from build123d import *

# Parameters (mm, degrees)
SKETCH_1_W          = 20
SKETCH_1_H          = 20
SKETCH_1_W_2        = 18
SKETCH_1_H_2        = 18
EXTRUDE_1_DEPTH     = 396
SKETCH_2_R          = 1.45
CUT_EXTRUDE_1_DEPTH = 397.630810704
SKETCH_3_R          = 1.45
CUT_EXTRUDE_2_DEPTH = 397.630810704


with BuildPart() as part:
    # 草图1 → 凸台-拉伸1 (new body)
    with BuildSketch(Plane(origin=(0, 0, 0), x_dir=(0, 0, -1), z_dir=(1, 0, 0))):
        Rectangle(SKETCH_1_W, SKETCH_1_H)
        Rectangle(SKETCH_1_W_2, SKETCH_1_H_2, mode=Mode.SUBTRACT)
    extrude(amount=EXTRUDE_1_DEPTH)

    # 草图2 → 切除-拉伸1 (cut, through all)
    with BuildSketch(Plane(origin=(0, 0, -10), x_dir=(-1, 0, 0), z_dir=(0, 0, -1))):
        with Locations((-380, -12.5)):
            Circle(SKETCH_2_R)
        with Locations(Location((-390.825317547, -6.25, 0), (0, 0, 90))):
            Circle(SKETCH_2_R)
        with Locations(Location((-390.825317547, 6.25, 0), (0, 0, 90))):
            Circle(SKETCH_2_R)
        with Locations((-380, 12.5)):
            Circle(SKETCH_2_R)
        with Locations(Location((-369.174682453, 6.25, 0), (0, 0, 90))):
            Circle(SKETCH_2_R)
        with Locations(Location((-369.174682453, -6.25, 0), (0, 0, 90))):
            Circle(SKETCH_2_R)
        with Locations(Location((-380, 0, 0), (0, 0, 90))):
            Circle(SKETCH_2_R)
    extrude(amount=-CUT_EXTRUDE_1_DEPTH, mode=Mode.SUBTRACT)

    # 草图3 → 切除-拉伸2 (cut, through all)
    with BuildSketch(Plane.XY.offset(10)):
        with Locations((10, 5)):
            Circle(SKETCH_3_R)
        with Locations((20, 5)):
            Circle(SKETCH_3_R)
        with Locations((10, -5)):
            Circle(SKETCH_3_R)
        with Locations((20, -5)):
            Circle(SKETCH_3_R)
        with Locations(Location((369.174682453, 6.25, 0), (0, 0, 90))):
            Circle(SKETCH_3_R)
        with Locations(Location((380, 0, 0), (0, 0, 90))):
            Circle(SKETCH_3_R)
        with Locations(Location((369.174682453, -6.25, 0), (0, 0, 90))):
            Circle(SKETCH_3_R)
        with Locations(Location((390.825317547, -6.25, 0), (0, 0, 90))):
            Circle(SKETCH_3_R)
        with Locations(Location((390.825317547, 6.25, 0), (0, 0, 90))):
            Circle(SKETCH_3_R)
    extrude(amount=-CUT_EXTRUDE_2_DEPTH, mode=Mode.SUBTRACT)


solid = part.part
Can you work these out from the model? Positions are in its coordinate system, mm. A direction names the side the tool comes from. Give positions to 0.01 mm unless a question says otherwise; leave off trailing zeros. Loops run counter-clockwise (first coordinate to the right, second up) from the corner with the lowest first, then second, coordinate; pieces in that order, holes last. Notation, with made-up numbers: (87, -0.5) -> (92, -0.5) arc R11 ccw to (92, 17.5) -> close; hole circle Ø9 at (64, 40.5). An arc over 180 degrees is marked (long way). Write item = value, one per line.
1) Will this pin go through, and if not, where does the flat tip stop? pin 1 (2.5 mm diameter, centred on x = 380, y = 0, fed in from -Z).
Check result:
pin_1 = through
2) Suppose I cut it at A-A on x = 152. Write out the boundary of the cut face in (y, z).
Check result:
outline = (-10, -10) -> (10, -10) -> (10, 10) -> (-10, 10) -> close; hole (-9, -9) -> (9, -9) -> (9, 9) -> (-9, 9) -> close
3) Suppose I cut it at B-B on z = -3.75. Write out the boundary of the cut face in (x, y).
Check result:
outline = (0, -10) -> (396, -10) -> (396, -9) -> (0, -9) -> close; (0, 9) -> (396, 9) -> (396, 10) -> (0, 10) -> close
4) Thinking about a two-plate mould opening in Y: for faces 3 (the flat face through (195, 10, 0)), 4 (the flat face through (195, -9, 0)), 5 (the flat face through (195, 0, -10)), which applies, released by +Y, released by -Y, zero draft, split by the parting line, or undercut?
Check result:
face_3 = released by +Y
face_4 = undercut
face_5 = zero draft
5) I need wall thicknesses on L1, parallel to Y at x = 208, z = -3; L2, parallel to Y at x = 380, z = 9.2. Which ranges of each line are inside material? Lowest first, please. Write a range as from..to.
Check result:
L1 = -10..-9, 9..10
L2 = -10..-1.45, 1.45..10
6) For faces 1 (the flat face through (396, -9.6, 0.8)), 2 (the flat face through (195, 0, 9)), which set-ups out of +Z, -Z, +X, -X, +Y, -Y let a thin tool reach every point of the face, with its end or its side?
Check result:
face_1 = +Z, -Z, +X, +Y, -Y
face_2 = +X, -X
